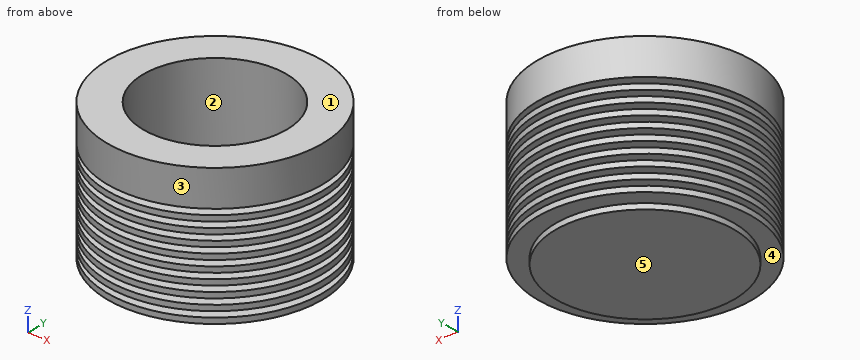
```python
from build123d import *

# Parameters (mm, degrees)
ESQUISSE1_R                = 38.1
BOSS_EXTRU_1_DEPTH         = 50.8
ESQUISSE2_OUTSIDE_W        = 102.028
ESQUISSE2_OUTSIDE_H        = 102.028
ESQUISSE2_OUTSIDE_R        = 31.75
ENL_V_MAT_EXTRU_3_DEPTH    = 2
R_P_TITION_LIN_AIRE1_COUNT = 10
R_P_TITION_LIN_AIRE1_PITCH = 4
ESQUISSE5_R                = 25.4
ENL_V_MAT_EXTRU_5_DEPTH    = 38.1


with BuildPart() as part:
    # Esquisse1 → Boss.-Extru.1 (new body)
    with BuildSketch(Plane.XY):
        Circle(ESQUISSE1_R)
    extrude(amount=BOSS_EXTRU_1_DEPTH)

    # Esquisse2 outside → Enlèv. mat.-Extru.3 (cut)
    with BuildSketch(Plane(origin=(0, 0, 0), x_dir=(-1, 0, 0), z_dir=(0, 0, -1))):
        Rectangle(ESQUISSE2_OUTSIDE_W, ESQUISSE2_OUTSIDE_H)
        Circle(ESQUISSE2_OUTSIDE_R, mode=Mode.SUBTRACT)
    enl_v_mat_extru_3 = extrude(amount=-ENL_V_MAT_EXTRU_3_DEPTH, mode=Mode.SUBTRACT)

    # Répétition linéaire1: Enlèv. mat.-Extru.3 ×10
    with Locations(*[(0, 0, i * R_P_TITION_LIN_AIRE1_PITCH) for i in range(1, R_P_TITION_LIN_AIRE1_COUNT)]):
        add(enl_v_mat_extru_3, mode=Mode.SUBTRACT)

    # Esquisse5 → Enlèv. mat.-Extru.5 (cut)
    with BuildSketch(Plane.XY.offset(50.8)):
        Circle(ESQUISSE5_R)
    extrude(amount=-ENL_V_MAT_EXTRU_5_DEPTH, mode=Mode.SUBTRACT)


solid = part.part
```
The model under review builds one solid part; all positions refer to its coordinate system, in mm. Face numbers are marked on the shaded views. A direction names the side the tool comes from. Round coordinates to 2 decimals unless told otherwise and drop trailing zeros. Order: outer loops, then holes, each group sorted by start corner. A loop starts at its lowest first (then second) coordinate and runs counter-clockwise, first axis right, second up.
Item 1: For pin 1 (8 mm diameter, centred on x = -16.5, z = 39.5, fed in from +Y); pin 2 (23 mm diameter, centred on x = -9.5, y = 2, fed in from +Z); pin 3 (2 mm diameter, centred on x = -22, z = 44, fed in from -Y), all flat-tipped, find the tip position at first contact; note any pin that passes through.
Working result:
pin 1: stops at y = 35.99
pin 2: stops at z = 12.7
pin 3: stops at y = -31.79
Item 2: Add section C-C, the plane z = 44.5. State the section outline as (x, y) points, and give its area (3 significant figures).
Working result:
outline: circle Ø76.2 at (0, 0); hole circle Ø50.8 at (0, 0)
area: 2,530 mm2
Item 3: Add section B-B, the plane z = 17. State the section outline as (x, y) points.
Working result:
outline: circle Ø63.5 at (0, 0); hole circle Ø50.8 at (0, 0)
Item 4: To check wall thickness, follow probe 1 along Y at (x, z) = (0, 34.5); probe 2 along Y at (x, z) = (0, 37); probe 3 along Z at (x, y) = (-8, -3). State the ranges of each line that lie inside material, in increasing order.
Working result:
probe 1: y = -38.1 to -25.4, 25.4 to 38.1
probe 2: y = -31.75 to -25.4, 25.4 to 31.75
probe 3: z = 0 to 12.7
Item 5: Machinability: for the marked faces 4 and 5, which of the approach directions +Z, -Z, +X, -X, +Y, -Y give a long, thin tool a straight path to every point of the face, cutting with its end or side? Answer none if there is none.
Working result:
face 4: -Z
face 5: -Z, +X, -X, +Y, -Y
Item 6: Draft analysis for pull direction X (two halves, no side actions). For the marked faces 1, 2 and 3, state which applies: released by +X, released by -X, zero draft, split by the parting line, or undercut.
Working result:
face 1: zero draft
face 2: undercut
face 3: split by the parting line
Item 7: Add section A-A, the plane z = 11. State the section outline as (x, y) points.
Working result:
outline: circle Ø76.2 at (0, 0)
